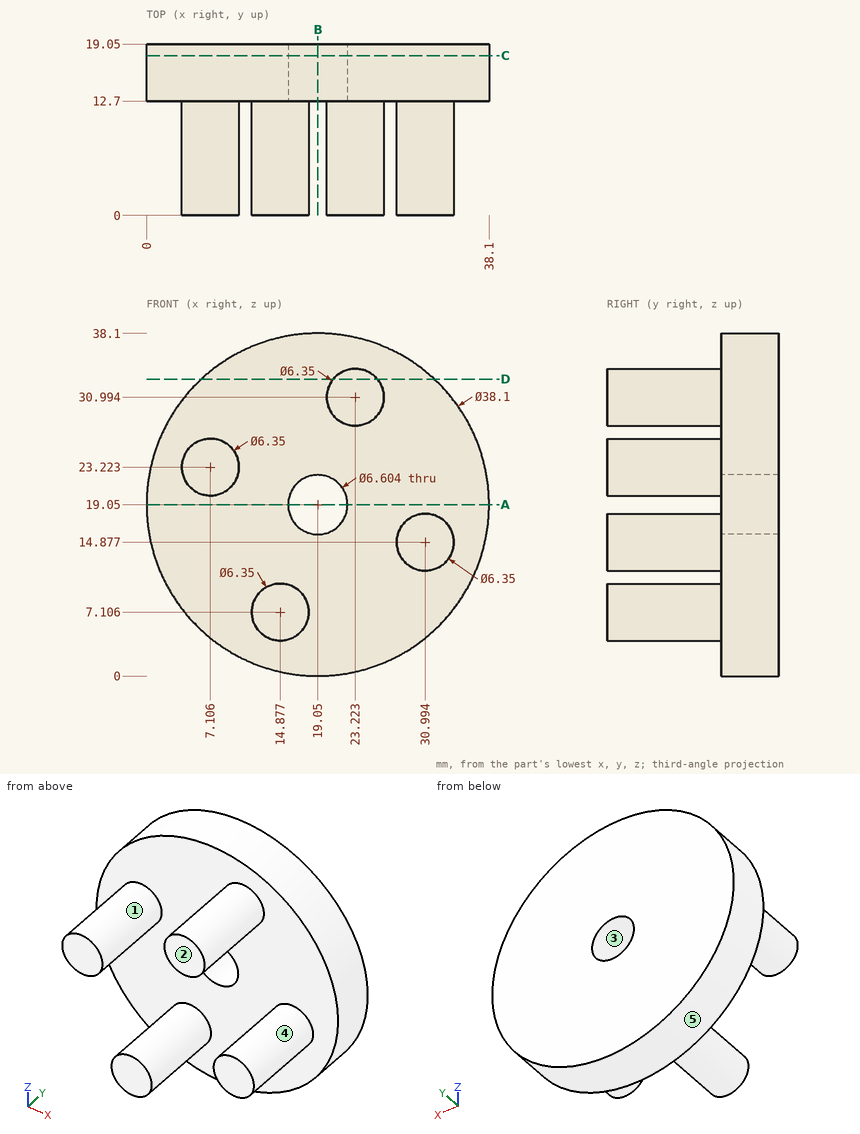
Print and shaded views of the part. All mm, measured from the part's lowest x, y and z. A direction names the side the tool comes from. Coordinates: 2 decimals unless noted, no trailing zeros. Order: outer loops, then holes, each group sorted by start corner. A loop starts at its lowest first (then second) coordinate and runs counter-clockwise, first axis right, second up. Notation, with made-up numbers: (-36.75, 13.5) -> (17.25, 13.5) arc R28 cw to (17.25, 32.5) -> close; hole circle Ø6 at (73, 45.5). An arc over 180 degrees is marked (long way). Answer as a JSON object with one key per item and string values. Group by question number.
1) Cut at A-A, the plane z = 19.05. Write the cut outline in (x, y).
2) Which spindle directions (+Z, -Z, +X, -X, +Y, -Y) get a long thin tool onto all of the face, cutting with end or side? Do the marked faces 4 and 5. Say none if no direction does.
3) Pull direction Z, two halves, no side cores. Call the marked faces 1, 2 and 3: +Z half, -Z half, draft (parallel to the pull), parting line (faces both ways), or undercut.
4) Cut at C-C, the plane y = 17.75. Write the cut outline in (x, z).
5) Cut at B-B, the plane x = 19.05. Write the cut outline in (y, z), then the cut area to 3 significant figures.
6) Cut at D-D, the plane z = 33. Write the cut outline in (x, y), then the cut area to 3 significant figures.
7) Flat gauge pins, fed straight in: pin 1 (3 mm diameter, centred on x = 28, y = 7.5, fed in from +Z); pin 2 (1.5 mm diameter, centred on x = 22, z = 5.5, fed in from -Y); pin 3 (10 mm diameter, centred on y = 6.5, z = 14.5, fed in from +X). Where does each tip first touch, or does it go through?
8) Drill centre lines: L1, parallel to Z at x = 19.05, y = 17; L2, parallel to Y at x = 27, z = 11; L3, parallel to X at y = 15.5, z = 20. Where is each one in solid material? Low to high.
Check values:
{
 "1": {"outline": "(0, 12.7) -> (15.75, 12.7) -> (15.75, 19.05) -> (0, 19.05) -> close; (22.35, 12.7) -> (38.1, 12.7) -> (38.1, 19.05) -> (22.35, 19.05) -> close"},
 "2": {"face 4": "-Y", "face 5": "+Y, -Y"},
 "3": {"face 1": "parting line", "face 2": "draft", "face 3": "undercut"},
 "4": {"outline": "circle Ø38.1 at (19.05, 19.05); hole circle Ø6.6 at (19.05, 19.05)"},
 "5": {"outline": "(12.7, 0) -> (19.05, 0) -> (19.05, 15.75) -> (12.7, 15.75) -> close; (12.7, 22.35) -> (19.05, 22.35) -> (19.05, 38.1) -> (12.7, 38.1) -> close", "area": "200 mm²"},
 "6": {"outline": "(6.08, 12.7) -> (20.76, 12.7) -> (20.76, 0) -> (25.68, 0) -> (25.68, 12.7) -> (32.02, 12.7) -> (32.02, 19.05) -> (6.08, 19.05) -> close", "area": "227 mm²"},
 "7": {"pin 1": "stops at z = 17.68", "pin 2": "stops at y = 12.7", "pin 3": "stops at x = 34.17"},
 "8": {"L1": "z = 0 to 15.75, 22.35 to 38.1", "L2": "y = 12.7 to 19.05", "L3": "x = 0.02 to 15.89, 22.21 to 38.08"}
}
